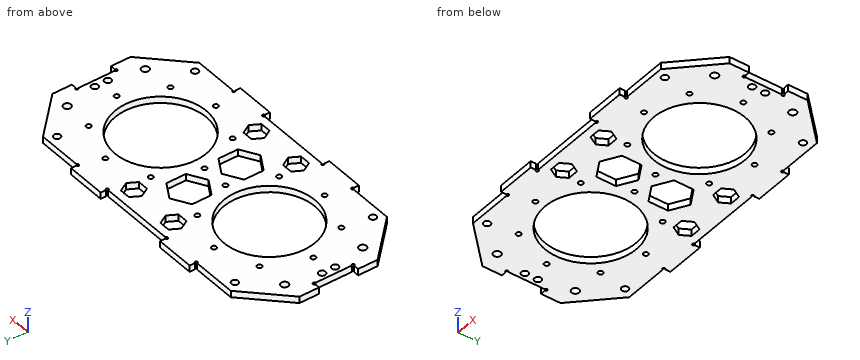
```python
from build123d import *

# Parameters (mm, degrees)
SKETCH_1_W          = 250
SKETCH_1_H          = 120
SKETCH_1_R          = 35
EXTRUDE_1_DEPTH     = 5
SKETCH_2_R          = 1.85
CUT_EXTRUDE_1_DEPTH = 10
CUT_EXTRUDE_2_DEPTH = 10
CUT_EXTRUDE_3_DEPTH = 10
SKETCH_7_W          = 30
SKETCH_7_H          = 5
EXTRUDE_2_DEPTH     = 5
SKETCH_8_R          = 1
CUT_EXTRUDE_4_DEPTH = 10
SKETCH_9_R          = 1
SKETCH_9_W          = 5
SKETCH_9_H          = 30
CUT_EXTRUDE_5_DEPTH = 5
SKETCH_10_R         = 2.6
SKETCH_10_R_2       = 2.85
CUT_EXTRUDE_6_DEPTH = 280.55321497


with BuildPart() as part:
    # 草图1 → 凸台-拉伸1 (new body)
    with BuildSketch(Plane.XY):
        with Locations((125, 60)):
            Rectangle(SKETCH_1_W, SKETCH_1_H)
        with Locations((70, 60)):
            Circle(SKETCH_1_R, mode=Mode.SUBTRACT)
        with Locations((180, 60)):
            Circle(SKETCH_1_R, mode=Mode.SUBTRACT)
    extrude(amount=EXTRUDE_1_DEPTH)

    # 草图2 → 切除-拉伸1 (cut)
    with BuildSketch(Plane.XY.offset(5)):
        with Locations((70, 102.5)):
            Circle(SKETCH_2_R)
        with Locations((70, 17.5)):
            Circle(SKETCH_2_R)
        with Locations((25.5, 60)):
            Circle(SKETCH_2_R)
        with Locations((38.533748237, 91.466251763)):
            Circle(SKETCH_2_R)
        with Locations((101.466251763, 91.466251763)):
            Circle(SKETCH_2_R)
        with Locations((114.5, 60)):
            Circle(SKETCH_2_R)
        with Locations((101.466251763, 28.533748237)):
            Circle(SKETCH_2_R)
        with Locations((38.533748237, 28.533748237)):
            Circle(SKETCH_2_R)
        with Locations((180, 102.5)):
            Circle(SKETCH_2_R)
        with Locations(Location((148.533748237, 91.466251763, 0), (0, 0, 180))):
            Circle(SKETCH_2_R)
        with Locations((135.5, 60)):
            Circle(SKETCH_2_R)
        with Locations((148.533748237, 28.533748237)):
            Circle(SKETCH_2_R)
        with Locations(Location((180, 17.5, 0), (0, 0, 180))):
            Circle(SKETCH_2_R)
        with Locations((211.466251763, 28.533748237)):
            Circle(SKETCH_2_R)
        with Locations((224.5, 60)):
            Circle(SKETCH_2_R)
        with Locations((211.466251763, 91.466251763)):
            Circle(SKETCH_2_R)
    extrude(amount=-CUT_EXTRUDE_1_DEPTH, mode=Mode.SUBTRACT)

    # 草图3 → 切除-拉伸2 (cut)
    with BuildSketch(Plane.XY.offset(5)):
        Polygon((0, 90), (30, 120), (0, 120), align=None)
        Polygon((30, 0), (0, 30), (0, 0), align=None)
        Polygon((250, 30), (220, 0), (250, 0), align=None)
        Polygon((250, 120), (220, 120), (250, 90), align=None)
    extrude(amount=-CUT_EXTRUDE_2_DEPTH, mode=Mode.SUBTRACT)

    # 草图4 → 切除-拉伸3 (cut)
    with BuildSketch(Plane(origin=(0, 0, 0), x_dir=(-1, 0, 0), z_dir=(0, 0, -1))):
        Polygon((-125, 65), (-112.009618943, 72.5), (-112.009618943, 87.5), (-125, 95), (-137.990381057, 87.5), (-137.990381057, 72.5), align=None)
        Polygon((-109, 100.143593539), (-113, 107.07179677), (-109, 114), (-101, 114), (-97, 107.07179677), (-101, 100.143593539), align=None)
        Polygon((-137, 107.07179677), (-141, 114), (-149, 114), (-153, 107.07179677), (-149, 100.143593539), (-141, 100.143593539), align=None)
        Polygon((-137.990381057, 47.5), (-125, 55), (-112.009618943, 47.5), (-112.009618943, 32.5), (-125, 25), (-137.990381057, 32.5), align=None)
        Polygon((-101, 19.856406461), (-109, 19.856406461), (-113, 12.92820323), (-109, 6), (-101, 6), (-97, 12.92820323), align=None)
        Polygon((-141, 19.856406461), (-137, 12.92820323), (-141, 6), (-149, 6), (-153, 12.92820323), (-149, 19.856406461), align=None)
    extrude(amount=-CUT_EXTRUDE_3_DEPTH, mode=Mode.SUBTRACT)

    # 草图7 → 凸台-拉伸2 (add)
    with BuildSketch(Plane.XY.offset(5)):
        with Locations((80, 122.5)):
            Rectangle(SKETCH_7_W, SKETCH_7_H)
        with Locations((170, 122.5)):
            Rectangle(SKETCH_7_W, SKETCH_7_H)
        with Locations((80, -2.5)):
            Rectangle(SKETCH_7_W, SKETCH_7_H)
        with Locations((170, -2.5)):
            Rectangle(SKETCH_7_W, SKETCH_7_H)
    extrude(amount=-EXTRUDE_2_DEPTH)

    # 草图8 → 切除-拉伸4 (cut)
    with BuildSketch(Plane.XY.offset(5)):
        with BuildLine():
            ThreePointArc((95, -1), (95.707106781, -0.707106781), (96, 0))
            Line((96, 0), (95, 0))
            Line((95, 0), (95, -1))
        make_face()
        with BuildLine():
            Line((95, 0), (96, 0))
            ThreePointArc((96, 0), (94.292893219, 0.707106781), (95, -1))
            Line((95, -1), (95, 0))
        make_face()
        with BuildLine():
            ThreePointArc((154, 0), (154.292893219, -0.707106781), (155, -1))
            Line((155, -1), (155, 0))
            Line((155, 0), (154, 0))
        make_face()
        with BuildLine():
            Line((155, 0), (155, -1))
            ThreePointArc((155, -1), (155.707106781, -0.707106781), (156, 0))
            ThreePointArc((156, 0), (155, 1), (154, 0))
            Line((154, 0), (155, 0))
        make_face()
        with BuildLine():
            ThreePointArc((185, -1), (185.707106781, -0.707106781), (186, 0))
            Line((186, 0), (185, 0))
            Line((185, 0), (185, -1))
        make_face()
        with BuildLine():
            Line((185, 0), (186, 0))
            ThreePointArc((186, 0), (184.292893219, 0.707106781), (185, -1))
            Line((185, -1), (185, 0))
        make_face()
        with BuildLine():
            ThreePointArc((156, 120), (155.707106781, 120.707106781), (155, 121))
            Line((155, 121), (155, 120))
            Line((155, 120), (154, 120))
            ThreePointArc((154, 120), (155, 119), (156, 120))
        make_face()
        with BuildLine():
            Line((155, 120), (155, 121))
            ThreePointArc((155, 121), (154.292893219, 120.707106781), (154, 120))
            Line((154, 120), (155, 120))
        make_face()
        with BuildLine():
            ThreePointArc((185, 121), (184.292893219, 119.292893219), (186, 120))
            Line((186, 120), (185, 120))
            Line((185, 120), (185, 121))
        make_face()
        with BuildLine():
            Line((185, 120), (186, 120))
            ThreePointArc((186, 120), (185.707106781, 120.707106781), (185, 121))
            Line((185, 121), (185, 120))
        make_face()
        with BuildLine():
            ThreePointArc((66, 120), (65.707106781, 120.707106781), (65, 121))
            Line((65, 121), (65, 120))
            Line((65, 120), (64, 120))
            ThreePointArc((64, 120), (65, 119), (66, 120))
        make_face()
        with BuildLine():
            Line((65, 120), (65, 121))
            ThreePointArc((65, 121), (64.292893219, 120.707106781), (64, 120))
            Line((64, 120), (65, 120))
        make_face()
        with BuildLine():
            ThreePointArc((95, 121), (94.292893219, 119.292893219), (96, 120))
            Line((96, 120), (95, 120))
            Line((95, 120), (95, 121))
        make_face()
        with BuildLine():
            Line((95, 120), (96, 120))
            ThreePointArc((96, 120), (95.707106781, 120.707106781), (95, 121))
            Line((95, 121), (95, 120))
        make_face()
        with Locations((65, 0)):
            Circle(SKETCH_8_R)
    extrude(amount=-CUT_EXTRUDE_4_DEPTH, mode=Mode.SUBTRACT)

    # 草图9 → 切除-拉伸5 (cut)
    with BuildSketch(Plane.XY.offset(5)):
        with Locations((5, 45)):
            Circle(SKETCH_9_R)
        with Locations((5, 75)):
            Circle(SKETCH_9_R)
        with Locations((2.5, 60)):
            Rectangle(SKETCH_9_W, SKETCH_9_H)
        with BuildLine():
            ThreePointArc((6, 75), (5, 76), (4, 75))
            Line((4, 75), (5, 75))
            Line((5, 75), (5, 74))
            ThreePointArc((5, 74), (5.707106781, 74.292893219), (6, 75))
        make_face()
        with BuildLine():
            Line((5, 75), (4, 75))
            ThreePointArc((4, 75), (4.292893219, 74.292893219), (5, 74))
            Line((5, 74), (5, 75))
        make_face()
        with BuildLine():
            ThreePointArc((6, 75), (5, 76), (4, 75))
            Line((4, 75), (5, 75))
            Line((5, 75), (5, 74))
            ThreePointArc((5, 74), (5.707106781, 74.292893219), (6, 75))
        make_face()
        with BuildLine():
            Line((5, 75), (4, 75))
            ThreePointArc((4, 75), (4.292893219, 74.292893219), (5, 74))
            Line((5, 74), (5, 75))
        make_face()
        with BuildLine():
            ThreePointArc((5, 46), (4.292893219, 45.707106781), (4, 45))
            Line((4, 45), (5, 45))
            Line((5, 45), (5, 46))
        make_face()
        with BuildLine():
            Line((5, 45), (4, 45))
            ThreePointArc((4, 45), (5, 44), (6, 45))
            ThreePointArc((6, 45), (5.707106781, 45.707106781), (5, 46))
            Line((5, 46), (5, 45))
        make_face()
        with BuildLine():
            ThreePointArc((5, 46), (4.292893219, 45.707106781), (4, 45))
            Line((4, 45), (5, 45))
            Line((5, 45), (5, 46))
        make_face()
        with BuildLine():
            Line((5, 45), (4, 45))
            ThreePointArc((4, 45), (5, 44), (6, 45))
            ThreePointArc((6, 45), (5.707106781, 45.707106781), (5, 46))
            Line((5, 46), (5, 45))
        make_face()
        with BuildLine():
            ThreePointArc((245, 74), (245.707106781, 74.292893219), (246, 75))
            Line((246, 75), (245, 75))
            Line((245, 75), (245, 74))
        make_face()
        with BuildLine():
            Line((245, 75), (246, 75))
            ThreePointArc((246, 75), (244.292893219, 75.707106781), (245, 74))
            Line((245, 74), (245, 75))
        make_face()
        with Locations((245, 45)):
            Circle(SKETCH_9_R)
        with Locations((245, 75)):
            Circle(SKETCH_9_R)
        with Locations((247.5, 60)):
            Rectangle(SKETCH_9_W, SKETCH_9_H)
        with BuildLine():
            ThreePointArc((245, 74), (245.707106781, 74.292893219), (246, 75))
            Line((246, 75), (245, 75))
            Line((245, 75), (245, 74))
        make_face()
        with BuildLine():
            Line((245, 75), (246, 75))
            ThreePointArc((246, 75), (244.292893219, 75.707106781), (245, 74))
            Line((245, 74), (245, 75))
        make_face()
        with BuildLine():
            ThreePointArc((245, 46), (244.292893219, 44.292893219), (246, 45))
            Line((246, 45), (245, 45))
            Line((245, 45), (245, 46))
        make_face()
        with BuildLine():
            Line((245, 45), (246, 45))
            ThreePointArc((246, 45), (245.707106781, 45.707106781), (245, 46))
            Line((245, 46), (245, 45))
        make_face()
        with BuildLine():
            ThreePointArc((245, 46), (244.292893219, 44.292893219), (246, 45))
            Line((246, 45), (245, 45))
            Line((245, 45), (245, 46))
        make_face()
        with BuildLine():
            Line((245, 45), (246, 45))
            ThreePointArc((246, 45), (245.707106781, 45.707106781), (245, 46))
            Line((245, 46), (245, 45))
        make_face()
    extrude(amount=-CUT_EXTRUDE_5_DEPTH, mode=Mode.SUBTRACT)

    # 草图10 → 切除-拉伸6 (cut, through all)
    with BuildSketch(Plane.XY.offset(5)):
        with Locations((10, 55)):
            Circle(SKETCH_10_R)
        with Locations((15, 30)):
            Circle(SKETCH_10_R_2)
        with Locations((35, 7)):
            Circle(SKETCH_10_R)
        with Locations((215, 7)):
            Circle(SKETCH_10_R)
        with Locations((235, 30)):
            Circle(SKETCH_10_R_2)
        with Locations((240, 55)):
            Circle(SKETCH_10_R)
        with Locations(Location((10, 65, 0), (0, 0, 180))):
            Circle(SKETCH_10_R)
        with Locations(Location((15, 90, 0), (0, 0, 180))):
            Circle(SKETCH_10_R_2)
        with Locations(Location((35, 113, 0), (0, 0, 180))):
            Circle(SKETCH_10_R)
        with Locations((215, 113)):
            Circle(SKETCH_10_R)
        with Locations((235, 90)):
            Circle(SKETCH_10_R_2)
        with Locations((240, 65)):
            Circle(SKETCH_10_R)
    extrude(amount=-CUT_EXTRUDE_6_DEPTH, mode=Mode.SUBTRACT)


solid = part.part
```
Build history of the part. All positions in model axes, mm. Give positions to 0.01 mm unless a question says otherwise; leave off trailing zeros. Loops run counter-clockwise (first coordinate to the right, second up) from the corner with the lowest first, then second, coordinate; pieces in that order, holes last. Notation, with made-up numbers: (70, -16) -> (128, -16) arc R22 ccw to (128, 18) -> close; hole circle Ø10 at (-1.5, 24). An arc over 180 degrees is marked (long way). One line per question, with ' | ' between items.
Q1. Cut at B-B, the plane z = 4.2. Count the separate pieces of the cut face and the enclosed holes in it, plus the area to 3 significant figures.
Filled sheet:
separate pieces: 1 | enclosed holes: 36 | area: 18,500 mm²
Q2. Drill centre lines: line 1 along X through (y, z) = (84.5, 2.35) (3 decimals); line 2 along Y through (x, z) = (94.5, 3.9) (3 decimals); line 3 along X through (y, z) = (77, 0.35). Where is each one in solid material? Low to high. Write a range as [from, to].
Filled sheet:
line 1: x = [0, 45.005], [94.995, 112.01], [137.99, 155.005], [204.995, 250] | line 2: y = [-5, -0.866], [0.866, 35.005], [84.995, 119.134], [120.866, 125] | line 3: x = [0, 39.41], [100.59, 112.01], [137.99, 149.41], [210.59, 250]
Q3. Drop flat-ended pins along their axis: pin 1 (3.5 mm diameter, centred on x = 135.5, y = 60, fed in from +Z); pin 2 (2.5 mm diameter, centred on x = 54.5, z = 2.5, fed in from +Y); pin 3 (2.5 mm diameter, centred on x = 103.5, z = 1.5, fed in from -Y). Give the stop position or say it passes through.
Filled sheet:
pin 1: passes through | pin 2: stops at y = 120 | pin 3: stops at y = 0
Q4. Cut at A-A, the plane x = 194. Write the cut outline in (y, z).
Filled sheet:
outline: (0, 0) -> (27.92, 0) -> (27.92, 5) -> (0, 5) -> close; (92.08, 0) -> (120, 0) -> (120, 5) -> (92.08, 5) -> close
